```python
from build123d import *

# Parameters (mm, degrees)
SKETCH1_W           = 11.1
SKETCH1_H           = 2.4
BOSS_EXTRUDE1_DEPTH = 20
CUT_EXTRUDE1_REACH  = 32.727
SKETCH2_R           = 4.05
SKETCH4_W           = 11.1
SKETCH4_H           = 3.65
BOSS_EXTRUDE3_DEPTH = 4.4
BOSS_EXTRUDE4_DEPTH = 1.9
BOSS_EXTRUDE5_DEPTH = 5.9


with BuildPart() as part:
    # Sketch1 → Boss-Extrude1 (new body)
    with BuildSketch(Plane.XY):
        with BuildLine():
            Line((-10.5, 0), (-3.5, 0))
            Line((-3.5, 0), (-3.5, -1.6))
            Line((-3.5, -1.6), (-15, -1.6))
            Line((-15, -1.6), (-18.031088913, 0.15))
            Line((-18.031088913, 0.15), (-18.031088913, 1.15))
            Line((-18.031088913, 1.15), (-15, 2.9))
            Line((-15, 2.9), (-12.5, 2.9))
            Line((-12.5, 2.9), (-10.55, 4.85))
            Line((-10.55, 4.85), (-10.55, 10.65))
            Line((-10.55, 10.65), (-8, 13.2))
            Line((-8, 13.2), (8, 13.2))
            Line((8, 13.2), (10.55, 10.65))
            Line((10.55, 10.65), (10.55, 4.85))
            Line((10.55, 4.85), (12.5, 2.9))
            Line((12.5, 2.9), (15, 2.9))
            Line((15, 2.9), (18.031088913, 1.15))
            Line((18.031088913, 1.15), (18.031088913, 0.15))
            Line((18.031088913, 0.15), (15, -1.6))
            Line((15, -1.6), (3.5, -1.6))
            Line((3.5, -1.6), (3.5, 0))
            Line((3.5, 0), (10.5, 0))
            Line((10.5, 0), (10.5, 1.7))
            Line((10.5, 1.7), (5.4, 1.7))
            Line((5.4, 1.7), (5.4, 4.8))
            ThreePointArc((5.4, 4.8), (4.814213562, 6.214213562), (3.4, 6.8))
            Line((3.4, 6.8), (-3.4, 6.8))
            ThreePointArc((-3.4, 6.8), (-4.814213562, 6.214213562), (-5.4, 4.8))
            Line((-5.4, 4.8), (-5.4, 1.7))
            Line((-5.4, 1.7), (-10.5, 1.7))
            Line((-10.5, 1.7), (-10.5, 0))
        make_face()
        with Locations((0, 10)):
            Rectangle(SKETCH1_W, SKETCH1_H, mode=Mode.SUBTRACT)
    extrude(amount=BOSS_EXTRUDE1_DEPTH)

    # Cut-Extrude1: up to this face of the body (flat: up to its plane)
    cut_extrude1_end = Plane(part.part.faces().sort_by_distance((7, 0, 10))[0])
    # Sketch2 → Cut-Extrude1 (cut, up to the picked face)
    with BuildSketch(Plane(origin=(0, 13.2, 0), x_dir=(1, 0, 0), z_dir=(0, 1, 0)), mode=Mode.PRIVATE) as cut_extrude1_sk1:
        with Locations(Location((0, -10, 0), (0, 0, 270))):
            Circle(SKETCH2_R)
    cut_extrude1_tool1 = split(extrude(cut_extrude1_sk1.sketch, amount=-CUT_EXTRUDE1_REACH, mode=Mode.PRIVATE), bisect_by=cut_extrude1_end, keep=Keep.BOTH, mode=Mode.PRIVATE)
    add(cut_extrude1_tool1.solids().sort_by(Axis((0, 13.2, 10), (0, -1, 0)))[0], mode=Mode.SUBTRACT)

    # Sketch4 → Boss-Extrude3 (add)
    with BuildSketch(Plane(origin=(0, 13.2, 0), x_dir=(1, 0, 0), z_dir=(0, 1, 0))):
        with Locations((0, -1.825)):
            Rectangle(SKETCH4_W, SKETCH4_H)
    extrude(amount=-BOSS_EXTRUDE3_DEPTH)

    # Sketch5 → Boss-Extrude4 (add)
    with BuildSketch(Plane(origin=(0, 0, 0), x_dir=(-1, 0, 0), z_dir=(0, 0, -1))):
        Polygon((-10.5, 1.7), (-10.5, -1.6), (10.5, -1.6), (10.5, 1.7), (5.4, 1.7), (5.4, 4.6), (-5.4, 4.6), (-5.4, 1.7), align=None)
    extrude(amount=-BOSS_EXTRUDE4_DEPTH)

    # Sketch6 → Boss-Extrude5 (add)
    with BuildSketch(Plane.XY.offset(20)):
        Polygon((-3.5, -1.6), (-3.5, 0), (-10.5, 0), (-10.5, 1.7), (-5.4, 1.7), (-5.4, 4.6), (5.4, 4.6), (5.4, 1.7), (10.5, 1.7), (10.5, 0), (3.5, 0), (3.5, -1.6), align=None)
    extrude(amount=-BOSS_EXTRUDE5_DEPTH)


solid = part.part
```
Input: part model. Units: mm. Frame: model coordinates. A direction names the side the tool comes from. Coordinates: 2 decimals unless noted, no trailing zeros. Loops run counter-clockwise (first coordinate to the right, second up) from the corner with the lowest first, then second, coordinate; pieces in that order, holes last. Notation, with made-up numbers: (-40, 20.5) -> (-22, 20.5) arc R16 ccw to (-22, 32.5) -> close; hole circle Ø8 at (58, 83). An arc over 180 degrees is marked (long way). Use a Markdown table: item, result.
1) Cut plane D-D (y = 12.25). Return the cut outline in (x, z), then the cut area to 3 significant figures.
Results found:
| item | result |
|---|---|
| outline | (-8.95, 0) -> (8.95, 0) -> (8.95, 20) -> (-8.95, 20) -> close; hole circle Ø8.1 at (0, 10) |
| area | 306 mm2 |
2) Pull-direction query (Z, two-part tool) for faces 1 (the flat face through (0, 2, 1.9)), 2 (the flat face through (0, 10, 3.65)), 3 (the flat face through (-11.5, 3.9, 9.9)); classes: released by +Z, released by -Z, zero draft, split by the parting line, or undercut.
Results found:
| item | result |
|---|---|
| face 1 | undercut |
| face 2 | released by +Z |
| face 3 | zero draft |
3) Material intervals for line 1 along Y through (x, z) = (3.5, 19); line 2 along X through (y, z) = (7.9, 10); line 3 along Z through (x, y) = (0, 8.35), sorted ascending. Write a range as from..to.
Results found:
| item | result |
|---|---|
| line 1 | y = -1.6..4.6, 6.8..8.8, 11.2..13.2 |
| line 2 | x = -10.55..-4.05, 4.05..10.55 |
| line 3 | z = 0..5.95, 14.05..20 |
4) Cut plane C-C (y = 6). Return the cut outline in (x, z).
Results found:
| item | result |
|---|---|
| outline | (-10.55, 0) -> (-5, 0) -> (-5, 20) -> (-10.55, 20) -> close; (5, 0) -> (10.55, 0) -> (10.55, 20) -> (5, 20) -> close |
5) Access query for faces 4 (the flat face through (-3, 8.8, 14)), 5 (the flat face through (4, -1.6, 10)), 6 (the flat face through (-5.4, 3, 8)), 7 (the cylindrical face through (5, 6, 10)). Directions: +Z, -Z, +X, -X, +Y, -Y. A direction counts if a zero-diameter tool reaches every point of the face in a straight line with its end or side. Return the directions, or none.
Results found:
| item | result |
|---|---|
| face 4 | +Z |
| face 5 | +Z, -Z, +X, -X, -Y |
| face 6 | none |
| face 7 | +Z, -Z |
6) Contact query for flat-ended pins moving along their axis: pin 1 (6.5 mm diameter, centred on y = 9, z = 8.5, fed in from -X); pin 2 (1.2 mm diameter, centred on x = -13.5, z = 14.5, fed in from +Y); pin 3 (1.3 mm diameter, centred on y = -1, z = 7.5, fed in from +X); pin 4 (1 mm diameter, centred on x = 10, y = 1, fed in from -Z). Output: stop coordinate, or through.
Results found:
| item | result |
|---|---|
| pin 1 | stops at x = -10.55 |
| pin 2 | stops at y = 2.9 |
| pin 3 | stops at x = 17.17 |
| pin 4 | stops at z = 0 |
7) Cut plane B-B (z = 17.5). Return the cut outline in (x, y).
Results found:
| item | result |
|---|---|
| outline | (-18.03, 0.15) -> (-15, -1.6) -> (15, -1.6) -> (18.03, 0.15) -> (18.03, 1.15) -> (15, 2.9) -> (12.5, 2.9) -> (10.55, 4.85) -> (10.55, 10.65) -> (8, 13.2) -> (-8, 13.2) -> (-10.55, 10.65) -> (-10.55, 4.85) -> (-12.5, 2.9) -> (-15, 2.9) -> (-18.03, 1.15) -> close; hole (-5.55, 8.8) -> (5.55, 8.8) -> (5.55, 11.2) -> (-5.55, 11.2) -> close; hole (-5.4, 4.6) -> (5.4, 4.6) -> (5.4, 4.8) arc R2 ccw to (3.4, 6.8) -> (-3.4, 6.8) arc R2 ccw to (-5.4, 4.8) -> close |
8) Cut plane A-A (x = 0). Return the cut outline in (y, z), then the cut area to 3 significant figures.
Results found:
| item | result |
|---|---|
| outline | (-1.6, 0) -> (4.6, 0) -> (4.6, 1.9) -> (-1.6, 1.9) -> close; (-1.6, 14.1) -> (4.6, 14.1) -> (4.6, 20) -> (-1.6, 20) -> close; (6.8, 0) -> (13.2, 0) -> (13.2, 5.95) -> (11.2, 5.95) -> (11.2, 3.65) -> (8.8, 3.65) -> (8.8, 5.95) -> (6.8, 5.95) -> close; (6.8, 14.05) -> (8.8, 14.05) -> (8.8, 20) -> (6.8, 20) -> close; (11.2, 14.05) -> (13.2, 14.05) -> (13.2, 20) -> (11.2, 20) -> close |
| area | 105 mm2 |
